Part print with two shaded views. Sizes in mm from the minimum x, y, z corner. Round coordinates to 2 decimals unless told otherwise and drop trailing zeros. Order: outer loops, then holes, each group sorted by start corner. A loop starts at its lowest first (then second) coordinate and runs counter-clockwise, first axis right, second up. Notation, with made-up numbers: M 85,34.25 L 119,34.25 A25 ccw 119,54.25 Z; hole C 67.5,-28 d2. An arc over 180 degrees is marked long. Put each result on its own line as item: value.
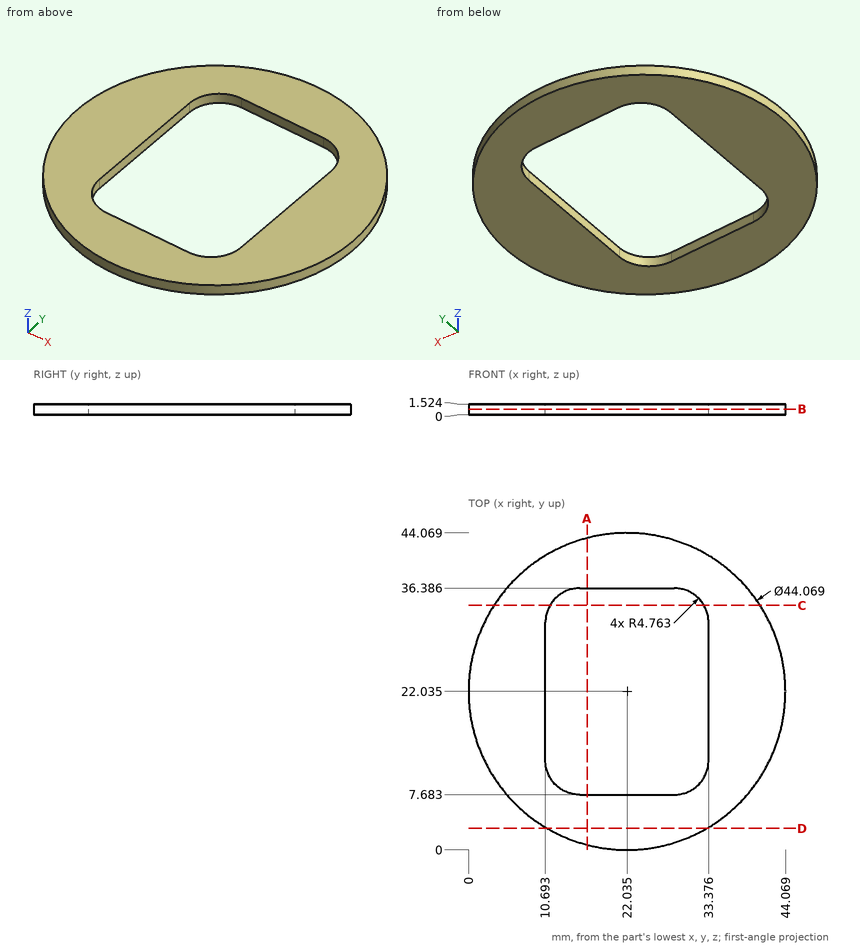
Item 1: Band-saw the part on C-C on y = 34. Give the cut face in (x, z) (1 decimal).
Answers below:
outline: M 3.5,0 L 11.3,0 L 11.3,1.5 L 3.5,1.5 Z; M 32.7,0 L 40.5,0 L 40.5,1.5 L 32.7,1.5 Z
Item 2: Band-saw the part on B-B on z = 0.8. Give the cut face in (x, y) (1 decimal).
Answers below:
outline: C 22,22 d44.1; hole M 10.7,12.4 A4.8 ccw 15.5,7.7 L 28.6,7.7 A4.8 ccw 33.4,12.4 L 33.4,31.6 A4.8 ccw 28.6,36.4 L 15.5,36.4 A4.8 ccw 10.7,31.6 Z
Item 3: Pin check, flat tips, straight feed: P1, Ø0.5, axis at x = 21, z = 1, coming from the -Y side; P2, Ø0.5, axis at x = 19.5, z = 0.5, coming from the +Y side. Stop position of each tip, or through.
Answers below:
P1: y = 0.01
P2: y = 43.95
Item 4: Probe line 1 along Y through (x, z) = (26.5, 1.2) (1 decimal); line 2 along X through (y, z) = (17, 1.05) (1 decimal); line 3 along Y through (x, z) = (25, 0.4) (1 decimal). List the from-to ranges inside material, lowest first. Write a range as [from, to].
Answers below:
line 1: [0.5, 7.7], [36.4, 43.6]
line 2: [0.6, 10.7], [33.4, 43.5]
line 3: [0.2, 7.7], [36.4, 43.9]
Item 5: Band-saw the part on A-A on x = 16.5. Give the cut face in (y, z) (1 decimal).
Answers below:
outline: M 0.7,0 L 7.7,0 L 7.7,1.5 L 0.7,1.5 Z; M 36.4,0 L 43.4,0 L 43.4,1.5 L 36.4,1.5 Z
Item 6: Band-saw the part on D-D on y = 3. Give the cut face in (x, z) (1 decimal).
Answers below:
outline: M 10.9,0 L 33.1,0 L 33.1,1.5 L 10.9,1.5 Z
